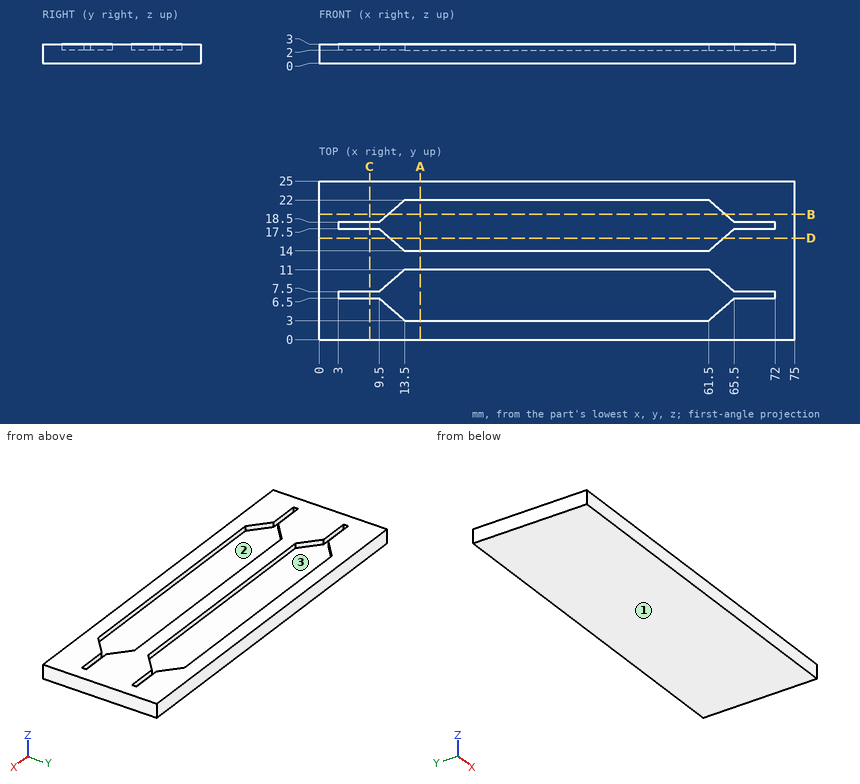
Geometry check sheet. Reference: drawing and pictorial views, mm from the part's lowest x, y, z. Coordinates: 2 decimals unless noted, no trailing zeros. Write each loop counter-clockwise with the first axis right and the second up, starting at its lowest first coordinate (ties: lowest second). Pieces come first, ordered by that corner, then holes. Notation, with made-up numbers: M 18,39 L 23,39 A23 cw 23,57 Z; hole C 46,-22 d1. An arc over 180 degrees is marked long. Use one line per item in the form item = value.
Item 1: Sectioned sample at B-B, the plane y = 19.75. Record the cut outline in (x, z).
Answer below:
outline = M 0,0 L 75,0 L 75,3 L 64.07,3 L 64.07,2 L 10.93,2 L 10.93,3 L 0,3 Z
Item 2: Material ranges on L1, parallel to Y at x = 14, z = 2.95; L2, parallel to Z at x = 25, y = 17; L3, parallel to X at y = 20, z = 2.4, recorded low to high. Write a range as from..to.
Answer below:
L1 = 0..3, 11..14, 22..25
L2 = 0..2
L3 = 0..11.21, 63.79..75
Item 3: Sectioned sample at D-D, the plane y = 16. Record the cut outline in (x, z), and give its area (3 significant figures).
Answer below:
outline = M 0,0 L 75,0 L 75,3 L 63.79,3 L 63.79,2 L 11.21,2 L 11.21,3 L 0,3 Z
area = 172 mm^2
Item 4: Release check for a two-part mould opening along X. For the marked faces 1, 2 and 3 record: pulls with the +X half, pulls with the -X half, needs draft (parallel to the pull), parting line crosses it, or undercut.
Answer below:
face_1 = needs draft
face_2 = undercut
face_3 = undercut
Item 5: Sectioned sample at C-C, the plane x = 8. Record the cut outline in (y, z), and give its area (3 significant figures).
Answer below:
outline = M 0,0 L 25,0 L 25,3 L 18.5,3 L 18.5,2 L 17.5,2 L 17.5,3 L 7.5,3 L 7.5,2 L 6.5,2 L 6.5,3 L 0,3 Z
area = 73.0 mm^2
Item 6: Sectioned sample at A-A, the plane x = 16. Record the cut outline in (y, z), and give its area (3 significant figures).
Answer below:
outline = M 0,0 L 25,0 L 25,3 L 22,3 L 22,2 L 14,2 L 14,3 L 11,3 L 11,2 L 3,2 L 3,3 L 0,3 Z
area = 59.0 mm^2
Item 7: Gauge pin test, flat end, axial feed: pin 1 Ø6 at (x, y) = (57, 7.5) entering from +Z. Record the tip position at first contact, or that the pin passes through.
Answer below:
pin_1 = 2
